CAD build for the part. Positions are in the model's coordinates, mm. A direction names the side the tool comes from. Coordinates: 2 decimals unless noted, no trailing zeros. Loops run counter-clockwise (first coordinate to the right, second up) from the corner with the lowest first, then second, coordinate; pieces in that order, holes last. Notation, with made-up numbers: (49, 85) -> (72, 85) arc R14 ccw to (72, 109) -> close; hole circle Ø1 at (70.5, 60). An arc over 180 degrees is marked (long way). Answer as a JSON object with one key per item and string values. Group by question number.
from build123d import *

# Parameters (mm, degrees)
F8_W      = 60.2088514067
F8_H      = 41.021
F9_DEPTH  = 11.176
F6_R      = 2.3749
F7_R      = 2.3749
F10_DEPTH = 12.192
F11_W     = 38.481
F11_H     = 26.162
F12_DEPTH = 9.1694
F13_DEPTH = 1.9558
F3_R      = 1.4605
F5_R      = 1.4605
F14_DEPTH = 12.192
F15_DEPTH = 1.9558


with BuildPart() as f9:
    # F8 (on Top) → F9 (new body)
    with BuildSketch(Plane.XY):
        Rectangle(F8_W, F8_H)
    extrude(amount=F9_DEPTH)

    # F6 (on face) + F7 (on face) → F10 (cut)
    with BuildSketch(Plane.XY):
        with Locations((-23.9141, -15.367)):
            Circle(F6_R)
    with BuildSketch(Plane.XY):
        with Locations((23.9141, 15.367)):
            Circle(F7_R)
    extrude(amount=F10_DEPTH, mode=Mode.SUBTRACT)

    # F11 (on face) → F12 (cut)
    with BuildSketch(Plane.XY.offset(11.176)):
        Rectangle(F11_W, F11_H)
    extrude(amount=-F12_DEPTH, mode=Mode.SUBTRACT)

    # F2 (on Top) → F13 (cut)
    with BuildSketch(Plane.XY):
        Polygon((-26.0612942775, 12.7635), (-23.0550314258, 12.7635), (-21.5519, 15.367), (-23.0550314258, 17.9705), (-26.0612942775, 17.9705), (-27.5644257033, 15.367), align=None)
    extrude(amount=F13_DEPTH, mode=Mode.SUBTRACT)

    # F3 (on face) + F5 (on face) → F14 (cut)
    with BuildSketch(Plane.XY):
        with Locations((-24.5581628517, 15.367)):
            Circle(F3_R)
    with BuildSketch(Plane.XY):
        with Locations((24.5581628517, -15.367)):
            Circle(F5_R)
    extrude(amount=F14_DEPTH, mode=Mode.SUBTRACT)

    # F4 (on face) → F15 (cut)
    with BuildSketch(Plane.XY):
        Polygon((23.0550314258, -17.9705), (26.0612942775, -17.9705), (27.5644257033, -15.367), (26.0612942775, -12.7635), (23.0550314258, -12.7635), (21.5519, -15.367), align=None)
    extrude(amount=F15_DEPTH, mode=Mode.SUBTRACT)


solid = f9.part
Item 1: Pull direction Y, two halves, no side cores. Call faces 4 (the flat face through (0, -20.51, 6)), 5 (the cylindrical face through (26.18, 16.08, 5.51)), 6 (the flat face through (30.104, 0, 6)): +Y half, -Y half, draft (parallel to the pull), parting line (faces both ways), or undercut.
Item 2: Band-saw the part on C-C, the plane z = 7.25. List the corners of the cut face in (x, y).
Item 3: 3-axis set-ups, long thin cutter, end or side, ignore diameter. For faces 1 (the flat face through (0, 13.081, 7)), 2 (the cylindrical face through (25.907, -15.926, 6.501)), 3 (the flat face through (25, -17.97, 1)): which of +Z, -Z, +X, -X, +Y, -Y reach the whole face in a straight line?
Item 4: Band-saw the part on D-D, the plane y = 12. List the corners of the cut face in (x, z).
Item 5: Band-saw the part on B-B, the plane x = 13. List the corners of the cut face in (y, z).
Item 6: Drill centre lines: L1, parallel to X at y = 9.5, z = 7.75; L2, parallel to Y at x = -18, z = 6.25; L3, parallel to X at y = 15.5, z = 9. Where is each one in solid material? Low to high.
Item 7: Flat gauge pins, fed straight in: P1, Ø1.6, axis at x = 25, y = -14, coming from the -Z side; P2, Ø8, axis at x = -3, y = 5.5, coming from the +Z side. Where does each tip first touch, or does it go through?
Item 8: Band-saw the part on A-A, the plane z = 1. List the corners of the cut face in (x, y), and give its area (3 significant figures).
Reply:
{
 "1": {"face 4": "-Y half", "face 5": "undercut", "face 6": "draft"},
 "2": {"outline": "(-30.1, -20.51) -> (30.1, -20.51) -> (30.1, 20.51) -> (-30.1, 20.51) -> close; hole circle Ø4.75 at (-23.91, -15.37); hole circle Ø2.92 at (-24.56, 15.37); hole (-19.24, -13.08) -> (19.24, -13.08) -> (19.24, 13.08) -> (-19.24, 13.08) -> close; hole circle Ø4.75 at (23.91, 15.37); hole circle Ø2.92 at (24.56, -15.37)"},
 "3": {"face 1": "+Z", "face 2": "+Z, -Z", "face 3": "-Z"},
 "4": {"outline": "(-30.1, 0) -> (30.1, 0) -> (30.1, 11.18) -> (19.24, 11.18) -> (19.24, 2.01) -> (-19.24, 2.01) -> (-19.24, 11.18) -> (-30.1, 11.18) -> close"},
 "5": {"outline": "(-20.51, 0) -> (20.51, 0) -> (20.51, 11.18) -> (13.08, 11.18) -> (13.08, 2.01) -> (-13.08, 2.01) -> (-13.08, 11.18) -> (-20.51, 11.18) -> close"},
 "6": {"L1": "-30.1 to -19.24, 19.24 to 30.1", "L2": "-20.51 to -13.08, 13.08 to 20.51", "L3": "-30.1 to -26.01, -23.1 to 21.54, 26.29 to 30.1"},
 "7": {"P1": "z = 1.96", "P2": "z = 2.01"},
 "8": {"outline": "(-30.1, -20.51) -> (30.1, -20.51) -> (30.1, 20.51) -> (-30.1, 20.51) -> close; hole (-27.56, 15.37) -> (-26.06, 12.76) -> (-23.06, 12.76) -> (-21.55, 15.37) -> (-23.06, 17.97) -> (-26.06, 17.97) -> close; hole circle Ø4.75 at (-23.91, -15.37); hole circle Ø4.75 at (23.91, 15.37); hole (21.55, -15.37) -> (23.06, -17.97) -> (26.06, -17.97) -> (27.56, -15.37) -> (26.06, -12.76) -> (23.06, -12.76) -> close", "area": "2,390 mm²"}
}
